Autodesk Inventor part; units mm, degrees
ref_plane "YZ Plane" through (0, 0, 0) normal (1, 0, 0) x (0, 1, 0)
ref_plane "XZ Plane" through (0, 0, 0) normal (0, 1, 0) x (-1, 0, 0)
ref_plane "XY Plane" through (0, 0, 0) normal (0, 0, 1) x (1, 0, 0)
sketch "Sketch1" plane through (0, 0, 0) normal (0, 1, 0) x (-1, 0, 0)
  circle A0 centre (0, 0) radius 1.465
  circle A1 centre (0, 0) radius 2.75
  line L0 (0.7073, -1.225) -> (-0.7073, -1.225)
  line L1 (-0.7073, -1.225) -> (-1.4145, 0)
  line L2 (-1.4145, 0) -> (-0.7073, 1.225)
  line L3 (-0.7073, 1.225) -> (0.7073, 1.225)
  line L4 (0.7073, 1.225) -> (1.4145, 0)
  line L5 (1.4145, 0) -> (0.7073, -1.225)
  dimension "d0" = 2.93
  dimension "d1" = 5.5
  dimension "d8" = 2.45
extrude "Extrusion1" add sketch "Sketch1" along normal blind 3 contours A0 | A1 | L0 L1 L2 L3 L4 L5
extrude "Extrusion2" add sketch "Sketch1" against normal blind 8 contours A0 | L0 L1 L2 L3 L4 L5
extrude "Extrusion3" cut sketch "Sketch1" against normal blind 2 from surface at 3 contours L0 L1 L2 L3 L4 L5
fillet "Fillet1" radius 0.5 1 edges at (2.75, 3, 0)
thread "Thread2"
equation "\"d4\" = length"
equation "\"length\" = 8"
properties part number "M3x16"
Part model, mm, in its own coordinate system. A direction names the side the tool comes from. Give positions to 0.01 mm unless a question says otherwise; leave off trailing zeros. Order: outer loops, then holes, each group sorted by start corner. A loop starts at its lowest first (then second) coordinate and runs counter-clockwise, first axis right, second up. Notation, with made-up numbers: (61, 64.5) - (113, 64.5) arc R21 cw to (113, 79.5) - close; hole circle Ø2 at (6, -17). An arc over 180 degrees is marked (long way). Use one line per item in the form item = value.
Item 1: Slice it at B-B on x = 0. Give the cut face in (y, z) (3 decimals).
Solution:
outline = (-8, -1.465) - (0, -1.465) - (0, -2.75) - (2.5, -2.75) arc R0.5 ccw to (3, -2.25) - (3, -1.225) - (1, -1.225) - (1, 1.225) - (3, 1.225) - (3, 2.25) arc R0.5 ccw to (2.5, 2.75) - (0, 2.75) - (0, 1.465) - (-8, 1.465) - close
Item 2: Slice it at C-C on y = -6.75. Give the cut face in (x, z) (3 decimals), and give its area (3 significant figures).
Solution:
outline = circle Ø2.93 at (0, 0)
area = 6.74 mm2
Item 3: Pin check, flat tips, straight feed: pin 1 Ø2 at (x, z) = (0.5, 0) entering from +Y; pin 2 Ø3 at (x, y) = (2, -0.5) entering from -Z; pin 3 Ø1.5 at (x, y) = (1, -2) entering from +Z. Stop position of each tip, or through.
Solution:
pin_1 = 3
pin_2 = -2.69
pin_3 = 1.44
Item 4: Two-plate mould, pull along Z, no slides. Class faces 4 (the face through (1.056, 2.014, -0.621)), 5 (the face through (0.32, -3.94, -1.43)), 6 (the face through (0, -8, 0)): released by +Z, released by -Z, zero draft, split by the parting line, or undercut.
Solution:
face_4 = undercut
face_5 = split by the parting line
face_6 = zero draft
Item 5: Which spindle directions (+Z, -Z, +X, -X, +Y, -Y) get a long thin tool onto all of the face, cutting with end or side? Do faces 1 (the face through (-1.2, 0, -1.2)), 2 (the face through (0.596, 1.232, 2.685)), 3 (the face through (1.07, 2.01, 0.6)). Say none if no direction does.
Solution:
face_1 = -Y
face_2 = +Y, -Y
face_3 = +Y
Item 6: Probe probe 1 along Y at (x, z) = (0.15, -1.7); probe 2 along X at (y, z) = (-5.5, -0.1); probe 3 along Y at (x, z) = (-0.4, -0.95). List the from-to ranges inside material, lowest first. Write a range as from..to.
Solution:
probe_1 = 0..3
probe_2 = -1.46..1.46
probe_3 = -8..1
